from build123d import *

# Parameters (mm, degrees)
SKETCH1_W           = 15
SKETCH1_H           = 110
BOSS_EXTRUDE1_DEPTH = 3
CUT_EXTRUDE1_DEPTH  = 3
SKETCH3_W           = 15
SKETCH3_H           = 3
BOSS_EXTRUDE2_DEPTH = 30
CUT_EXTRUDE2_DEPTH  = 30


with BuildPart() as part:
    # Sketch1 → Boss-Extrude1 (new body)
    with BuildSketch(Plane.XY):
        Rectangle(SKETCH1_W, SKETCH1_H)
    extrude(amount=BOSS_EXTRUDE1_DEPTH)

    # Sketch2 → Cut-Extrude1 (cut)
    with BuildSketch(Plane.XY.offset(3)):
        with BuildLine():
            Line((2, 15), (2, -50))
            ThreePointArc((2, -50), (0, -52), (-2, -50))
            Line((-2, -50), (-2, 15))
            ThreePointArc((-2, 15), (0, 17), (2, 15))
        make_face()
    extrude(amount=-CUT_EXTRUDE1_DEPTH, mode=Mode.SUBTRACT)

    # Sketch3 → Boss-Extrude2 (add)
    with BuildSketch(Plane.XY.offset(3)):
        with Locations((0, 53.5)):
            Rectangle(SKETCH3_W, SKETCH3_H)
    extrude(amount=BOSS_EXTRUDE2_DEPTH)

    # Sketch4 → Cut-Extrude2 (cut)
    with BuildSketch(Plane(origin=(0, 55, 0), x_dir=(1, 0, 0), z_dir=(0, 1, 0))):
        with BuildLine():
            Line((2, -5), (2, -28))
            ThreePointArc((2, -28), (0, -30), (-2, -28))
            Line((-2, -28), (-2, -5))
            ThreePointArc((-2, -5), (0, -3), (2, -5))
        make_face()
    extrude(amount=-CUT_EXTRUDE2_DEPTH, mode=Mode.SUBTRACT)


solid = part.part
Verification items for the finished model (mm, model axes). A direction names the side the tool comes from. Coordinates: 2 decimals unless noted, no trailing zeros. Order: outer loops, then holes, each group sorted by start corner. A loop starts at its lowest first (then second) coordinate and runs counter-clockwise, first axis right, second up. Notation, with made-up numbers: M 30.25,84.25 L 45.25,84.25 A18 cw 45.25,112.25 Z; hole C 61.5,-14.5 d4. An arc over 180 degrees is marked long. Return JSON: item names as keys, results as strings.
1) Gauge pin test, flat ends, axial feed: pin 1 (4 mm diameter, centred on x = 3, z = 27.5, fed in from -Y); pin 2 (7.5 mm diameter, centred on x = 0, y = 0.5, fed in from +Z); pin 3 (2 mm diameter, centred on x = 0, y = -4, fed in from -Z). Record the tip position at first contact, or that the pin passes through.
Answer list:
{"pin 1": "y = 52", "pin 2": "z = 3", "pin 3": "through"}
2) Access from +Z, -Z, +X, -X, +Y, -Y to the whole of each face (thin tool, end or side, straight path). Record for faces 1 (the cylindrical face through (0, 54, 30)), 2 (the flat face through (-3, 52, 18)), 3 (the flat face through (-2, -18, 2)), 4 (the flat face through (-3, 55, 16)).
Answer list:
{"face 1": "+Y, -Y", "face 2": "+Z, +X, -X, -Y", "face 3": "+Z, -Z", "face 4": "+Z, -Z, +X, -X, +Y"}
3) Cross-section at B-B, the plane z = 16.5. Record the boundary of the cut face in (x, y), and give its area (3 significant figures).
Answer list:
{"outline": "M -7.5,52 L -2,52 L -2,55 L -7.5,55 Z; M 2,52 L 7.5,52 L 7.5,55 L 2,55 Z", "area": "33.0 mm2"}
4) Thickness scan on L1, parallel to Z at x = -4.25, y = 45; L2, parallel to Y at x = 3, z = 18. Record the ranges inside material, lowest first. Write a range as [from, to].
Answer list:
{"L1": "[0, 3]", "L2": "[52, 55]"}
5) Cross-section at A-A, the plane y = -20. Record the boundary of the cut face in (x, z).
Answer list:
{"outline": "M -7.5,0 L -2,0 L -2,3 L -7.5,3 Z; M 2,0 L 7.5,0 L 7.5,3 L 2,3 Z"}
6) Cross-section at D-D, the plane y = 47.5. Record the boundary of the cut face in (x, z), and give its area (3 significant figures).
Answer list:
{"outline": "M -7.5,0 L 7.5,0 L 7.5,3 L -7.5,3 Z", "area": "45.0 mm2"}
7) Cross-section at C-C, the plane x = 4.5. Record the boundary of the cut face in (y, z), and give its area (3 significant figures).
Answer list:
{"outline": "M -55,0 L 55,0 L 55,33 L 52,33 L 52,3 L -55,3 Z", "area": "420 mm2"}
8) Release check for a two-part mould opening along X. For faces 5 (the flat face through (-7.5, 12, 2)), 6 (the flat face through (2, 54, 16)), 7 (the flat face through (-3, 1, 0)), 8 (the cylindrical face through (0, -52, 2)) record: +X half, -X half, draft (parallel to the pull), parting line (faces both ways), or undercut.
Answer list:
{"face 5": "-X half", "face 6": "undercut", "face 7": "draft", "face 8": "undercut"}
